The model under review builds one solid part; all positions refer to its coordinate system, in mm. Face numbers are marked on the shaded views. A direction names the side the tool comes from. Coordinates: 2 decimals unless noted, no trailing zeros. Write each loop counter-clockwise with the first axis right and the second up, starting at its lowest first coordinate (ties: lowest second). Pieces come first, ordered by that corner, then holes.
1) Add section A-A, the plane y = 5. State the section outline as (x, z) points.
2) Machinability: for the marked faces 1, 2, 3, 4 and 5, which of the approach directions +Z, -Z, +X, -X, +Y, -Y give a long, thin tool a straight path to every point of the face, cutting with its end or side? Answer none if there is none.
3) Add section D-D, the plane x = 3.5. State the section outline as (y, z) points.
4) Mouldability with a two-part tool opening along Y and no side actions: class the marked faces 6, 7 and 8 as released by +Y, released by -Y, zero draft, split by the parting line, or undercut.
5) For P1, Ø0.6, axis at x = 5.5, y = 21.5, coming from the -Z side; P2, Ø1.6, axis at x = 5, y = 21.5, coming from the +Z side; P3, Ø0.7, axis at x = 5.5, y = 8.5, coming from the +Z side, all flat-tipped, find the tip position at first contact; note any pin that passes through.
6) Add section C-C, the plane z = -5.5. State the section outline as (x, y) points.
7) Add section B-B, the plane z = 0. State the section outline as (x, y) points.
8) For line 1 (X direction, y = 2, z = 0.5); line 2 (X direction, y = 14, z = -2.75); line 3 (Y direction, x = -2.25, z = -1.25), list the stretches that pass through material, from the lowest coordinate up.
from build123d import *

# Parameters (mm, degrees)
SKETCH1_W            = 13
SKETCH1_H            = 9
BOSS_EXTRUDE1_DEPTH  = 1.5
BOSS_EXTRUDE2_DEPTH  = 2
FILLET1_R            = 1
FILLET1_OF_MIRROR1_R = 1
FILLET2_START        = -4.5
FILLET2_DEPTH        = 4
FILLET2_START_2      = 0.5
FILLET2_2_DEPTH      = 4
FILLET2_3_DEPTH      = 1.695635927
FILLET2_START_3      = 2.821367992
FILLET2_4_DEPTH      = 1.678632008
FILLET2_START_4      = -0.5
FILLET2_5_DEPTH      = 1
FILLET2_6_DEPTH      = 1


with BuildPart() as part:
    # Sketch1 → Boss-Extrude1 (new body)
    with BuildSketch(Plane(origin=(0, 0, 0), x_dir=(1, 0, 0), z_dir=(0, 1, 0))):
        Rectangle(SKETCH1_W, SKETCH1_H)
    extrude(amount=BOSS_EXTRUDE1_DEPTH)

    # Sketch2 → Boss-Extrude2 (add)
    with BuildSketch(Plane.ZY.offset(6.5)):
        with BuildLine():
            Line((-4.5, 1.5), (4.5, 1.5))
            Line((4.5, 1.5), (4.5, 14.090918463))
            ThreePointArc((4.5, 14.090918463), (6.058811408, 20.2265006), (1.5, 24.618823416))
            Line((1.5, 24.618823416), (1.5, 20.243559577))
            ThreePointArc((1.5, 20.243559577), (2.230950643, 17.940661794), (0.5, 16.255005568))
            Line((0.5, 16.255005568), (0.5, 2.5))
            ThreePointArc((0.5, 2.5), (0, 2), (-0.5, 2.5))
            Line((-0.5, 2.5), (-0.5, 16.255005568))
            ThreePointArc((-0.5, 16.255005568), (-2.230950643, 17.940661794), (-1.5, 20.243559577))
            Line((-1.5, 20.243559577), (-1.5, 24.618823416))
            ThreePointArc((-1.5, 24.618823416), (-6.058811408, 20.2265006), (-4.5, 14.090918463))
            Line((-4.5, 14.090918463), (-4.5, 1.5))
        make_face()
    boss_extrude2 = extrude(amount=-BOSS_EXTRUDE2_DEPTH)

    # Fillet1
    fillet1_edges = [part.edges().sort_by_distance(p)[0] for p in [
        (-5.5, 14.090918463, -4.5),
        (-5.5, 24.618823416, -1.5),
        (-5.5, 24.618823416, 1.5),
        (-5.5, 14.090918463, 4.5),
    ]]
    fillet(fillet1_edges, radius=FILLET1_R)

    # Mirror1: Boss-Extrude2 across plane
    add(boss_extrude2.mirror(Plane(origin=(0, 0, 0), x_dir=(0, 0, 1), z_dir=(1, 0, 0))))

    # Fillet1 of Mirror1
    fillet1_of_mirror1_edges = [part.edges().sort_by_distance(p)[0] for p in [
        (5.5, 14.090918463, -4.5),
        (5.5, 24.618823416, -1.5),
        (5.5, 24.618823416, 1.5),
        (5.5, 14.090918463, 4.5),
    ]]
    fillet(fillet1_of_mirror1_edges, radius=FILLET1_OF_MIRROR1_R)

    # Fillet2: read off the stored shape, not the designer's step
    # Fillet2 outline → Fillet2 (add)
    with BuildSketch(Plane.XY.offset(FILLET2_START)):
        with BuildLine():
            ThreePointArc((4.5, 3.5), (3.914213562, 2.085786438), (2.5, 1.5))
            Line((2.5, 1.5), (4.5, 1.5))
            Line((4.5, 1.5), (4.5, 3.5))
        make_face()
        with BuildLine():
            ThreePointArc((-2.5, 1.5), (-3.914213562, 2.085786438), (-4.5, 3.5))
            Line((-4.5, 3.5), (-4.5, 1.5))
            Line((-4.5, 1.5), (-2.5, 1.5))
        make_face()
    extrude(amount=FILLET2_DEPTH)

    # Fillet2 2 outline → Fillet2 2 (add)
    with BuildSketch(Plane.XY.offset(FILLET2_START_2)):
        with BuildLine():
            ThreePointArc((4.5, 3.5), (3.914213562, 2.085786438), (2.5, 1.5))
            Line((2.5, 1.5), (4.5, 1.5))
            Line((4.5, 1.5), (4.5, 3.5))
        make_face()
        with BuildLine():
            ThreePointArc((-2.5, 1.5), (-3.914213562, 2.085786438), (-4.5, 3.5))
            Line((-4.5, 3.5), (-4.5, 1.5))
            Line((-4.5, 1.5), (-2.5, 1.5))
        make_face()
    extrude(amount=FILLET2_2_DEPTH)

    # Fillet2 3 outline → Fillet2 3 (add)
    with BuildSketch(Plane.YZ.offset(FILLET2_START)):
        with BuildLine():
            Line((1.5, -0.5), (2.5, -0.5))
            ThreePointArc((2.5, -0.5), (2, 0), (2.5, 0.5))
            Line((2.5, 0.5), (1.5, 0.5))
            Line((1.5, 0.5), (1.5, -0.5))
        make_face()
    extrude(amount=FILLET2_3_DEPTH)

    # Fillet2 4 outline → Fillet2 4 (add)
    with BuildSketch(Plane.YZ.offset(FILLET2_START_3)):
        with BuildLine():
            Line((1.5, -0.5), (2.5, -0.5))
            ThreePointArc((2.5, -0.5), (2, 0), (2.5, 0.5))
            Line((2.5, 0.5), (1.5, 0.5))
            Line((1.5, 0.5), (1.5, -0.5))
        make_face()
    extrude(amount=FILLET2_4_DEPTH)

    # Fillet2 5 outline → Fillet2 5 (cut)
    with BuildSketch(Plane.XY.offset(FILLET2_START_4)):
        with BuildLine():
            Line((-4.5, 4), (-4.5, 3.5))
            ThreePointArc((-4.5, 3.5), (-4.018013199, 2.19783414), (-2.804364073, 1.523295037))
            Line((-2.804364073, 1.523295037), (-2.804364073, 4))
            Line((-2.804364073, 4), (-4.5, 4))
        make_face()
        with BuildLine():
            Line((4.5, 4), (2.821367992, 4))
            Line((2.821367992, 4), (2.821367992, 1.525988193))
            ThreePointArc((2.821367992, 1.525988193), (4.02360362, 2.204379683), (4.5, 3.5))
            Line((4.5, 3.5), (4.5, 4))
        make_face()
    extrude(amount=FILLET2_5_DEPTH, mode=Mode.SUBTRACT)

    # Fillet2 6 outline → Fillet2 6 (add)
    with BuildSketch(Plane.XY.offset(FILLET2_START_4)):
        with BuildLine():
            ThreePointArc((-2.5, 1.5), (-2.652627117, 1.505832263), (-2.804364073, 1.523295037))
            Line((-2.804364073, 1.523295037), (-2.804364073, 1.5))
            Line((-2.804364073, 1.5), (-2.5, 1.5))
        make_face()
        with BuildLine():
            ThreePointArc((2.821367992, 1.525988193), (2.661208539, 1.506507636), (2.5, 1.5))
            Line((2.5, 1.5), (2.821367992, 1.499999997))
            Line((2.821367992, 1.499999997), (2.821367992, 1.525988193))
        make_face()
    extrude(amount=FILLET2_6_DEPTH)


solid = part.part
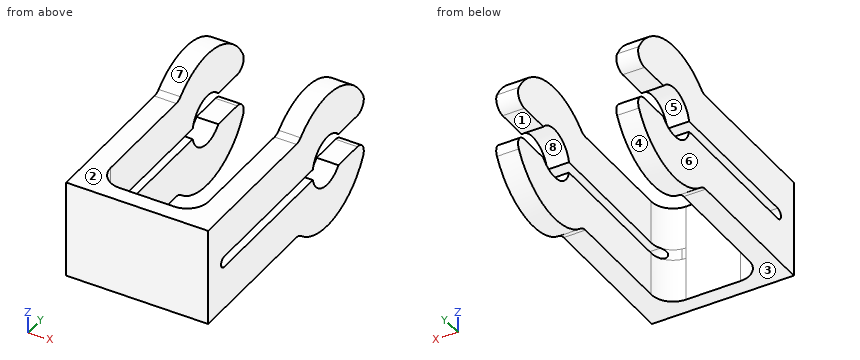
Geometry results:
1. outline: (-6.5, -4.5) - (-4.5, -4.5) - (-4.5, -0.5) - (-6.5, -0.5) - close; (-6.5, 0.5) - (-4.5, 0.5) - (-4.5, 4.5) - (-6.5, 4.5) - close; (4.5, -4.5) - (6.5, -4.5) - (6.5, -0.5) - (4.5, -0.5) - close; (4.5, 0.5) - (6.5, 0.5) - (6.5, 4.5) - (4.5, 4.5) - close
2. face 1: +X, -X, +Y
2. face 2: +Z, +X, -X, -Y
2. face 3: -Z, +X, -X, -Y
2. face 4: -Z, +X, -X
2. face 5: +X, -X
3. outline: (0, -4.5) - (1.77, -4.5) - (1.77, 4.5) - (0, 4.5) - close
4. face 6: zero draft
4. face 7: split by the parting line
4. face 8: undercut
5. P1: stops at z = -5.69
5. P2: stops at z = 5.9
5. P3: stops at z = 4.5
6. outline: (-6.5, 15.43) - (-4.5, 15.43) - (-4.5, 21.57) - (-6.5, 21.57) - close; (4.5, 15.43) - (6.5, 15.43) - (6.5, 21.57) - (4.5, 21.57) - close
7. outline: (-6.5, 0) - (6.5, 0) - (6.5, 2) - (3.82, 2) arc R2 cw to (2.5, 1.5) - (-2.5, 1.5) arc R2 cw to (-3.82, 2) - (-6.5, 2) - close
8. line 1: x = -6.5 to -3.82, 3.82 to 6.5
8. line 2: x = -6.5 to -4.5, 4.5 to 6.5
8. line 3: y = 0 to 1.5
